Verification items for the finished model (mm, model axes). Round coordinates to 2 decimals unless told otherwise and drop trailing zeros. Order: outer loops, then holes, each group sorted by start corner. A loop starts at its lowest first (then second) coordinate and runs counter-clockwise, first axis right, second up. Notation, with made-up numbers: (7, 12.5) -> (12, 12.5) arc R19 ccw to (12, 17.5) -> close; hole circle Ø10 at (37, 9.5). An arc over 180 degrees is marked (long way). Return JSON: item names as keys, results as strings. Group by question number.
Item 1: Sectioned sample at A-A on y = -5. Record the cut outline in (x, z).
Item 2: Sectioned sample at D-D on x = 59. Record the cut outline in (y, z).
Item 3: Depth check by flat-ended pin: pin 1 Ø8 at (y, z) = (5, -11) entering from -X. Enter the tip coordinate at first touch or a pass-through.
Item 4: Sectioned sample at B-B on x = 135. Record the cut outline in (y, z).
Item 5: Sectioned sample at C-C on z = 0. Record the cut outline in (x, y).
Item 6: Scan lines: probe 1 along X at (y, z) = (-13.7, 0); probe 2 along Y at (x, z) = (-31.5, 8). Record each from-to range of solid material in increasing order. Write a range as from..to.
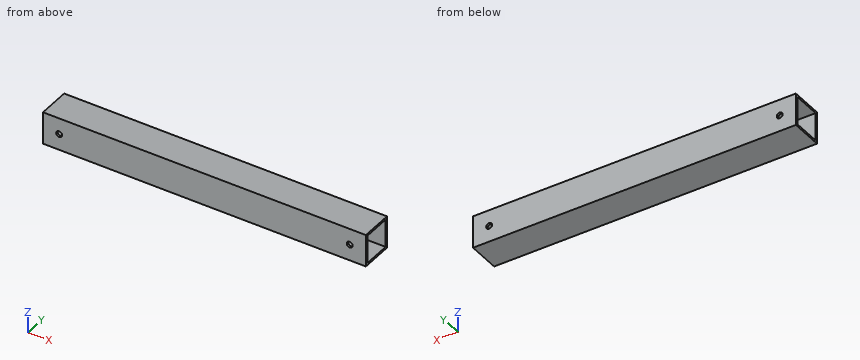
```python
from build123d import *

# Parameters (mm, degrees)
SKETCH1_W           = 30
SKETCH1_H           = 30
SKETCH1_W_2         = 26
SKETCH1_H_2         = 26
BOSS_EXTRUDE1_DEPTH = 150
SKETCH2_R           = 2.75
CUT_EXTRUDE1_DEPTH  = 152.492574075


with BuildPart() as part:
    # Sketch1 → Boss-Extrude1 (new, symmetric)
    with BuildSketch(Plane(origin=(0, 0, 0), x_dir=(0, 0, -1), z_dir=(1, 0, 0))):
        Rectangle(SKETCH1_W, SKETCH1_H)
        Rectangle(SKETCH1_W_2, SKETCH1_H_2, mode=Mode.SUBTRACT)
    extrude(amount=BOSS_EXTRUDE1_DEPTH, both=True)

    # Sketch2 → Cut-Extrude1 (cut, symmetric)
    with BuildSketch(Plane(origin=(0, 0, 0), x_dir=(1, 0, 0), z_dir=(0, 1, 0))):
        with Locations(Location((135, 0, 0), (0, 0, 270))):
            Circle(SKETCH2_R)
    cut_extrude1 = extrude(amount=CUT_EXTRUDE1_DEPTH, both=True, mode=Mode.SUBTRACT)

    # Mirror1: Cut-Extrude1 across plane
    add(cut_extrude1.mirror(Plane(origin=(0, 0, 0), x_dir=(0, 0, 1), z_dir=(1, 0, 0))), mode=Mode.SUBTRACT)


solid = part.part
```
Recorded:
{
 "1": {"outline": "(-150, -15) -> (150, -15) -> (150, -13) -> (-150, -13) -> close; (-150, 13) -> (150, 13) -> (150, 15) -> (-150, 15) -> close"},
 "2": {"outline": "(-15, -15) -> (15, -15) -> (15, 15) -> (-15, 15) -> close; hole (-13, -13) -> (13, -13) -> (13, 13) -> (-13, 13) -> close"},
 "3": {"pin 1": "x = -150"},
 "4": {"outline": "(-15, -15) -> (15, -15) -> (15, -2.75) -> (13, -2.75) -> (13, -13) -> (-13, -13) -> (-13, -2.75) -> (-15, -2.75) -> close; (-15, 2.75) -> (-13, 2.75) -> (-13, 13) -> (13, 13) -> (13, 2.75) -> (15, 2.75) -> (15, 15) -> (-15, 15) -> close"},
 "5": {"outline": "(-150, -15) -> (-137.75, -15) -> (-137.75, -13) -> (-150, -13) -> close; (-150, 13) -> (-137.75, 13) -> (-137.75, 15) -> (-150, 15) -> close; (-132.25, -15) -> (132.25, -15) -> (132.25, -13) -> (-132.25, -13) -> close; (-132.25, 13) -> (132.25, 13) -> (132.25, 15) -> (-132.25, 15) -> close; (137.75, -15) -> (150, -15) -> (150, -13) -> (137.75, -13) -> close; (137.75, 13) -> (150, 13) -> (150, 15) -> (137.75, 15) -> close"},
 "6": {"probe 1": "-150..-137.75, -132.25..132.25, 137.75..150", "probe 2": "-15..-13, 13..15"}
}
